Could you check a few things on this drawing? It's one solid part, dimensions in mm from its lowest x, y, z. Give positions to 0.01 mm unless a question says otherwise; leave off trailing zeros. Loops run counter-clockwise (first coordinate to the right, second up) from the corner with the lowest first, then second, coordinate; pieces in that order, holes last. Notation, with made-up numbers: (3, 2.25) - (16, 2.25) arc R27 ccw to (16, 20.25) - close; hole circle Ø7 at (69.25, 73). An arc over 180 degrees is marked (long way). Use a Markdown table: item, result.
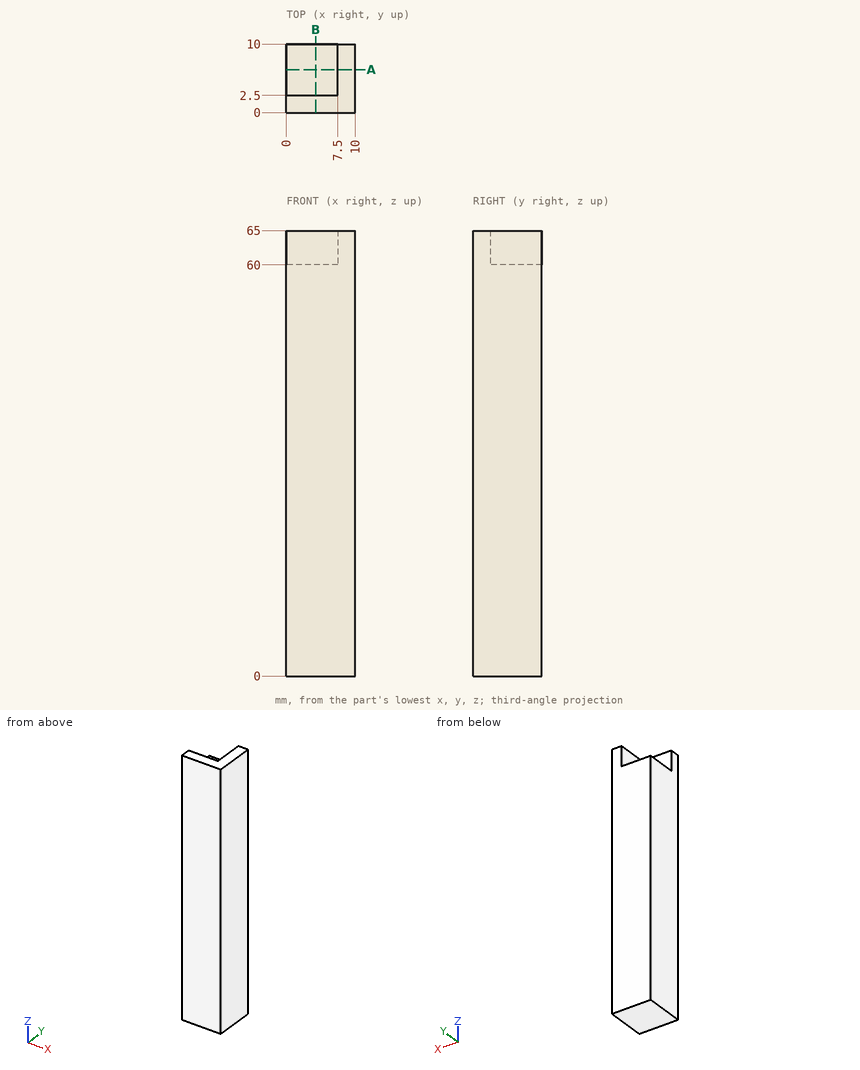
(1) Will these pins go through, and if not, where does the flat tip stop? pin 1 (2 mm diameter, centred on x = 5.5, z = 55, fed in from -Y); pin 2 (4 mm diameter, centred on x = 3.5, z = 63, fed in from +Y).
A:
| item | result |
|---|---|
| pin 1 | y = 0 |
| pin 2 | y = 2.5 |
(2) Suppose I cut it at A-A on y = 6.25. Write out the boundary of the cut face in (x, z).
A:
| item | result |
|---|---|
| outline | (0, 0) - (10, 0) - (10, 65) - (7.5, 65) - (7.5, 60) - (0, 60) - close |
(3) Suppose I cut it at B-B on x = 4.25. Write out the boundary of the cut face in (y, z).
A:
| item | result |
|---|---|
| outline | (0, 0) - (10, 0) - (10, 60) - (2.5, 60) - (2.5, 65) - (0, 65) - close |
(4) If I drill on line 1 (Z direction, x = 1.25, y = 4); line 2 (X direction, y = 3.75, z = 60.5); line 3 (Y direction, x = 1.75, z = 62.5), over which ranges is the centre line in solid material (lowest first)?
A:
| item | result |
|---|---|
| line 1 | 0 to 60 |
| line 2 | 7.5 to 10 |
| line 3 | 0 to 2.5 |
